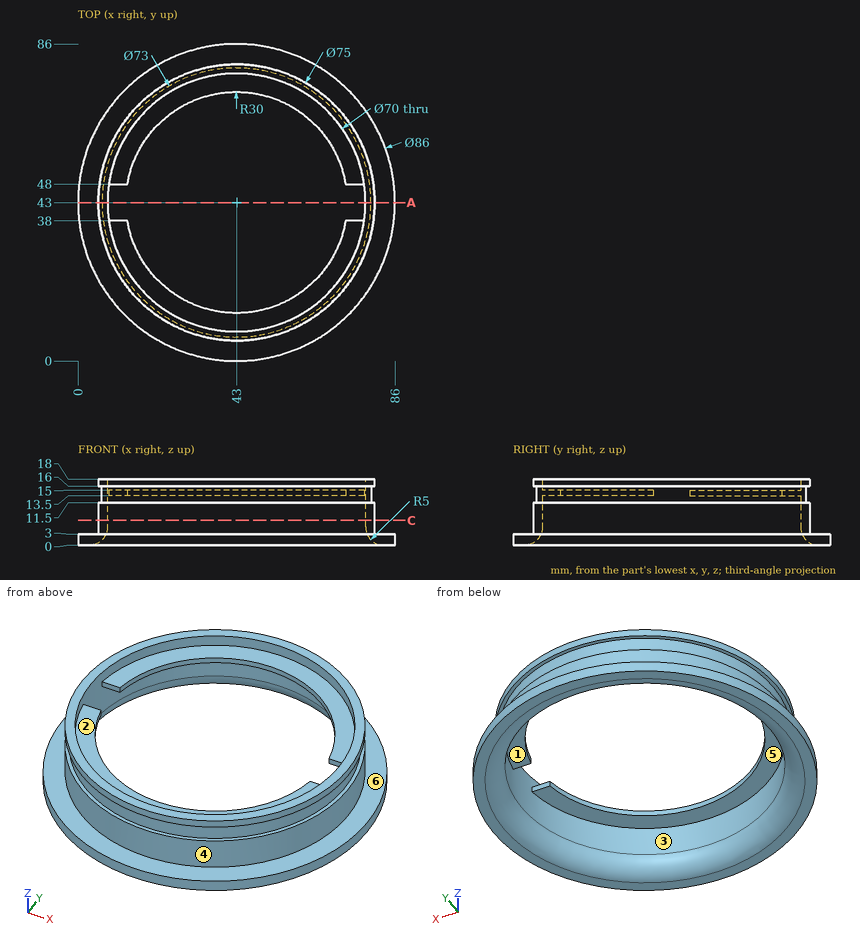
Can you work these out from the drawing? Everything is in mm from the part's minimum corner. A direction names the side the tool comes from. Coordinates: 2 decimals unless noted, no trailing zeros. Write each loop counter-clockwise with the first axis right and the second up, starting at its lowest first coordinate (ties: lowest second). Pieces come first, ordered by that corner, then holes. Notation, with made-up numbers: (-7, 14.25) -> (47, 14.25) arc R20 ccw to (47, 19.25) -> close; hole circle Ø4 at (88.25, -21.5). An arc over 180 degrees is marked (long way). Write item = value, one per line.
(1) Imagine slicing it at A-A (y = 43). Please give me the cut outline in (x, z), and give its area (3 significant figures).
Verdict:
outline = (0, 0) -> (3, 0) arc R5 ccw to (8, 5) -> (8, 18) -> (5.5, 18) -> (5.5, 16) -> (6.5, 16) -> (6.5, 11.5) -> (5.5, 11.5) -> (5.5, 3) -> (0, 3) -> close; (78, 5) arc R5 ccw to (83, 0) -> (86, 0) -> (86, 3) -> (80.5, 3) -> (80.5, 11.5) -> (79.5, 11.5) -> (79.5, 16) -> (80.5, 16) -> (80.5, 18) -> (78, 18) -> close
area = 103 mm^2
(2) Thinking about a two-plate mould opening in Y: for the marked faces 3, 4, 5 and 6, which applies, +Y half, -Y half, draft (parallel to the pull), parting line (faces both ways), or undercut?
Verdict:
face_3 = undercut
face_4 = parting line
face_5 = undercut
face_6 = draft
(3) Imagine slicing it at C-C (z = 6.75). Please give me the cut outline in (x, y).
Verdict:
outline = circle Ø75 at (43, 43); hole circle Ø70 at (43, 43)
(4) On a 3-axis mill with a long thin cutter (end or side, diameter ignored), from which of +Z, -Z, +X, -X, +Y, -Y can I reach the whole of each face in a straight line? I mean the marked faces 1 and 2. Say none if no direction works.
Verdict:
face_1 = -Z
face_2 = +Z
(5) If I drill on probe 1 along Y at (x, z) = (43, 8.5); probe 2 along Y at (x, z) = (26.5, 13.75); probe 3 along X at (y, z) = (38, 7.75), over which ranges is the centre line in solid material (lowest first)?
Verdict:
probe_1 = 5.5 to 8, 78 to 80.5
probe_2 = 10.44 to 17.95, 68.05 to 75.56
probe_3 = 5.83 to 8.36, 77.64 to 80.17
(6) For pin 1 (3 mm diameter, centred on x = 9.5, y = 66.5, fed in from -Z); pin 2 (1.6 mm diameter, centred on x = 10.5, z = 14, fed in from +Y); pin 3 (1.6 mm diameter, centred on x = 75, z = 14, fed in from -Y); pin 4 (15 mm diameter, centred on x = 27.5, y = 66.5, fed in from -Z), each with a flat end and sliding along its axis, tell me the tip position at first contact or that it passes through.
Verdict:
pin_1 = 0
pin_2 = 61.09
pin_3 = 24.06
pin_4 = 2.53
